Can you work these out from the model? Positions are in its coordinate system, mm. A direction names the side the tool comes from. Coordinates: 2 decimals unless noted, no trailing zeros. Loops run counter-clockwise (first coordinate to the right, second up) from the corner with the lowest first, then second, coordinate; pieces in that order, holes last.
```python
from build123d import *

# Parameters (mm, degrees)
BOSS_EXTRUDE3_DEPTH = 6.35
SKETCH5_W           = 7
SKETCH5_H           = 7
CUT_EXTRUDE3_DEPTH  = 3.175
SKETCH7_R           = 1.4224
SKETCH7_R_2         = 1.4732
CUT_EXTRUDE5_DEPTH  = 6.35
SKETCH8_W           = 3.175
SKETCH8_H           = 43.3
CUT_EXTRUDE6_DEPTH  = 10
SKETCH9_W           = 4
SKETCH9_H           = 4
CUT_EXTRUDE8_DEPTH  = 4
SKETCH10_W          = 5.175
SKETCH10_H          = 5.175
SKETCH10_W_2        = 5.18
CUT_EXTRUDE9_DEPTH  = 0.9


with BuildPart() as part:
    # Sketch2 → Boss-Extrude3 (new body)
    with BuildSketch(Plane(origin=(0, 0, 0), x_dir=(1, 0, 0), z_dir=(0, 1, 0))):
        with BuildLine():
            Line((-45, 25.825), (-45, -25.825))
            ThreePointArc((-45, -25.825), (-43.777170811, -28.777170811), (-40.825, -30))
            Line((-40.825, -30), (40.825, -30))
            ThreePointArc((40.825, -30), (43.777170811, -28.777170811), (45, -25.825))
            Line((45, -25.825), (45, 25.825))
            ThreePointArc((45, 25.825), (43.777170811, 28.777170811), (40.825, 30))
            Line((40.825, 30), (-40.825, 30))
            ThreePointArc((-40.825, 30), (-43.777170811, 28.777170811), (-45, 25.825))
        make_face()
        with BuildLine():
            Line((40.825, 21.65), (41.825, 21.65))
            Line((41.825, 21.65), (41.825, -21.65))
            Line((41.825, -21.65), (40.825, -21.65))
            ThreePointArc((40.825, -21.65), (37.872829189, -22.872829189), (36.65, -25.825))
            Line((36.65, -25.825), (36.65, -26.825))
            Line((36.65, -26.825), (-36.65, -26.825))
            Line((-36.65, -26.825), (-36.65, -25.825))
            ThreePointArc((-36.65, -25.825), (-37.872829189, -22.872829189), (-40.825, -21.65))
            Line((-40.825, -21.65), (-41.825, -21.65))
            Line((-41.825, -21.65), (-41.825, 21.65))
            Line((-41.825, 21.65), (-40.825, 21.65))
            ThreePointArc((-40.825, 21.65), (-37.872829189, 22.872829189), (-36.65, 25.825))
            Line((-36.65, 25.825), (-36.65, 26.825))
            Line((-36.65, 26.825), (36.65, 26.825))
            Line((36.65, 26.825), (36.65, 25.825))
            ThreePointArc((36.65, 25.825), (37.872829189, 22.872829189), (40.825, 21.65))
        make_face(mode=Mode.SUBTRACT)
    extrude(amount=BOSS_EXTRUDE3_DEPTH)

    # Sketch5 → Cut-Extrude3 (cut)
    with BuildSketch(Plane.ZY.offset(45)):
        with Locations((13.825, 0)):
            Rectangle(SKETCH5_W, SKETCH5_H)
    extrude(amount=-CUT_EXTRUDE3_DEPTH, mode=Mode.SUBTRACT)

    # Sketch7 → Cut-Extrude5 (cut)
    with BuildSketch(Plane.XZ):
        with Locations(Location((-40.825, -25.825, 0), (0, 0, 270))):
            Circle(SKETCH7_R)
        with Locations(Location((-40.825, 25.81356336, 0), (0, 0, 270))):
            Circle(SKETCH7_R_2)
        with Locations(Location((40.825, 25.825, 0), (0, 0, 270))):
            Circle(SKETCH7_R_2)
        with Locations(Location((40.825, -25.81487963, 0), (0, 0, 270))):
            Circle(SKETCH7_R_2)
    extrude(amount=-CUT_EXTRUDE5_DEPTH, mode=Mode.SUBTRACT)

    # Sketch8 → Cut-Extrude6 (cut)
    with BuildSketch(Plane(origin=(0, 6.35, 0), x_dir=(1, 0, 0), z_dir=(0, 1, 0))):
        with Locations((43.4125, 0)):
            Rectangle(SKETCH8_W, SKETCH8_H)
    extrude(amount=-CUT_EXTRUDE6_DEPTH, mode=Mode.SUBTRACT)

    # Sketch9 → Cut-Extrude8 (cut)
    with BuildSketch(Plane.XY.offset(30)):
        with Locations((-33.2866, 2)):
            Rectangle(SKETCH9_W, SKETCH9_H)
    extrude(amount=-CUT_EXTRUDE8_DEPTH, mode=Mode.SUBTRACT)

    # Sketch10 → Cut-Extrude9 (cut)
    with BuildSketch(Plane(origin=(0, 6.35, 0), x_dir=(1, 0, 0), z_dir=(0, 1, 0))):
        with Locations((-39.2375, 24.2375)):
            Rectangle(SKETCH10_W, SKETCH10_H)
        with Locations((-39.2375, -24.2375)):
            Rectangle(SKETCH10_W, SKETCH10_H)
        with Locations((39.24, -24.2375)):
            Rectangle(SKETCH10_W_2, SKETCH10_H)
        with Locations((39.24, 24.2375)):
            Rectangle(SKETCH10_W_2, SKETCH10_H)
    extrude(amount=-CUT_EXTRUDE9_DEPTH, mode=Mode.SUBTRACT)


solid = part.part
```
(1) I'm going to push flat-ended pins straight in: pin 1 (2.5 mm diameter, centred on x = -40, z = -24.5, fed in from +Y); pin 2 (0.8 mm diameter, centred on y = 3, z = -26.5, fed in from +X); pin 3 (1.1 mm diameter, centred on x = -41.5, y = 3.5, fed in from +Z); pin 4 (1.5 mm diameter, centred on y = 5.5, z = 7.5, fed in from +X) (3 decimals). Where does each tip first touch, or does it pass through?
Check values:
pin 1: stops at y = 5.45
pin 2: stops at x = 44.99
pin 3: stops at z = 30
pin 4: stops at x = -41.825
(2) I want a section at A-A on x = 17. Write out the boundary of the cut face in (y, z) (3 decimals).
Check values:
outline: (0, -30) - (6.35, -30) - (6.35, -26.825) - (0, -26.825) - close; (0, 26.825) - (6.35, 26.825) - (6.35, 30) - (0, 30) - close
(3) I want a section at C-C on z = 14. Write out the boundary of the cut face in (x, y) (3 decimals).
Check values:
outline: (-45, 3.5) - (-41.825, 3.5) - (-41.825, 6.35) - (-45, 6.35) - close
(4) I want a section at B-B on z = -16. Write out the boundary of the cut face in (x, y) (3 decimals), then the cut area to 3 significant figures.
Check values:
outline: (-45, 0) - (-41.825, 0) - (-41.825, 6.35) - (-45, 6.35) - close
area: 20.2 mm2
(5) Which directions (+Z, -Z, +X, -X, +Y, -Y) give clear straight access to the entire face, cutting with the end or side of a thin tool? Please do faces 1 (the cylindrical face through (-37.905, 2.687, -22.841)), 2 (the flat face through (-35.287, 2, 28)), 3 (the flat face through (-41, 0, 24)), 4 (the flat face through (-39, 5.45, 24)), 5 (the flat face through (-43, 2, 10.325)).
Check values:
face 1: +Y, -Y
face 2: +Z, -Y
face 3: +Z, -Z, +X, -X, -Y
face 4: +Y
face 5: +X, -X, -Y
(6) If we mould it in two halves opening along X, with no side actions, what happens to faces 6 (the flat face through (43, 3, -21.65)), 7 (the cylindrical face through (42.067, 3.131, -26.607)), 8 (the cylindrical face through (43.809, 3.131, -28.745))? For each: released by +X, released by -X, zero draft, split by the parting line, or undercut.
Check values:
face 6: zero draft
face 7: undercut
face 8: released by +X
(7) If I drill on probe 1 along Z at (x, y) = (-15, 4.5) (3 decimals); probe 2 along X at (y, z) = (1.75, -15) (3 decimals); probe 3 along Z at (x, y) = (39, 5), over which ranges is the centre line in solid material (lowest first)?
Check values:
probe 1: z = -30 to -26.825, 26.825 to 30
probe 2: x = -45 to -41.825
probe 3: z = -30 to -22.07, 22.07 to 30
